Could you check a few things on this model? Use its own coordinates, in mm. A direction names the side the tool comes from. Coordinates: 2 decimals unless noted, no trailing zeros. Write each loop counter-clockwise with the first axis right and the second up, starting at its lowest first coordinate (ties: lowest second). Pieces come first, ordered by that corner, then holes.
```python
from build123d import *

# Parameters (mm, degrees)
F1_DEPTH = 2.9972


with BuildPart() as f1:
    # F0 (on Right) → F1 (new body)
    with BuildSketch(Plane.YZ):
        Polygon((-25.4, 9.525), (-28.3972, 9.525), (-28.3972, -9.525), (-25.4, -9.525), (-25.4, -19.05), (0, -19.05), (25.4, -19.05), (25.4, -9.525), (28.3972, -9.525), (28.3972, 9.525), (25.4, 9.525), (25.4, 19.05), (0, 19.05), (-25.4, 19.05), align=None)
        Polygon((-12.7, -12.8778), (0, -12.8778), (12.7, -12.8778), (12.7, -15.875), (0, -15.875), (-12.7, -15.875), align=None, mode=Mode.SUBTRACT)
    extrude(amount=F1_DEPTH)


solid = f1.part
```
1. I want a section at A-A on y = -6. Please give me the cut outline in (x, z) (3 decimals).
Verdict:
outline: (0, -19.05) - (2.997, -19.05) - (2.997, -15.875) - (0, -15.875) - close; (0, -12.878) - (2.997, -12.878) - (2.997, 19.05) - (0, 19.05) - close
2. If we mould it in two halves opening along Z, with no side actions, what happens to faces 1 (the face through (1, -27, -9.525)), 2 (the face through (1, -12.7, -14)), 3 (the face through (1, -25.4, -14))? For each: pulls with the +Z half, pulls with the -Z half, needs draft (parallel to the pull), parting line crosses it, or undercut.
Verdict:
face 1: pulls with the -Z half
face 2: undercut
face 3: needs draft
3. I want a section at B-B on x = 1.8. Please give me the cut outline in (y, z) (3 decimals), plus the area to 3 significant figures.
Verdict:
outline: (-28.397, -9.525) - (-25.4, -9.525) - (-25.4, -19.05) - (25.4, -19.05) - (25.4, -9.525) - (28.397, -9.525) - (28.397, 9.525) - (25.4, 9.525) - (25.4, 19.05) - (-25.4, 19.05) - (-25.4, 9.525) - (-28.397, 9.525) - close; hole (-12.7, -15.875) - (12.7, -15.875) - (12.7, -12.878) - (-12.7, -12.878) - close
area: 1,970 mm2
4. For pin 1 (1.5 mm diameter, centred on x = 2, y = 27.5, fed in from +Z) (3 decimals); pin 2 (1.5 mm diameter, centred on x = 1.5, y = 27.5, fed in from -Z) (3 decimals); pin 3 (1.5 mm diameter, centred on x = 1.5, z = -14.5, fed in from -Y), each with a flat end and sliding along its axis, tell me the tip position at first contact or that it passes through.
Verdict:
pin 1: stops at z = 9.525
pin 2: stops at z = -9.525
pin 3: stops at y = -25.4
5. Please list where these lines run through material, in increasing order: line 1 along Z through (x, y) = (1.7, -11.5) (3 decimals); line 2 along Y through (x, z) = (0.2, -13.5); line 3 along Y through (x, z) = (0.6, 12).
Verdict:
line 1: z = -19.05 to -15.875, -12.878 to 19.05
line 2: y = -25.4 to -12.7, 12.7 to 25.4
line 3: y = -25.4 to 25.4
6. I want a section at C-C on z = 14. Please give me the cut outline in (x, y).
Verdict:
outline: (0, -25.4) - (3, -25.4) - (3, 25.4) - (0, 25.4) - close
7. On a 3-axis mill with a long thin cutter (end or side, diameter ignored), from which of +Z, -Z, +X, -X, +Y, -Y can I reach the whole of each face in a straight line? I mean faces 4 (the face through (1, 12.7, -14)), 5 (the face through (1, -25.4, 14)), 6 (the face through (1, 27, 9.525)). Say none if no direction works.
Verdict:
face 4: +X, -X
face 5: +Z, +X, -X, -Y
face 6: +Z, +X, -X, +Y
